from build123d import *

# Parameters (mm, degrees)
F0_W      = 42
F0_H      = 17
F1_DEPTH  = 7
F4_DEPTH  = 25
F5_W      = 42
F5_H      = 5.6745335534
F6_DEPTH  = 10
F7_R      = 1.675
F8_DEPTH  = 25
F9_DEPTH  = 25
F11_W     = 5.7
F11_H     = 7
F12_DEPTH = 5


with BuildPart() as f1:
    # F0 (on Top) → F1 (new body)
    with BuildSketch(Plane.XY):
        with Locations((21, 8.5)):
            Rectangle(F0_W, F0_H)
    extrude(amount=F1_DEPTH)

    # F3 (on face) → F4 (cut)
    with BuildSketch(Plane(origin=(0, 17, 0), x_dir=(-1, 0, 0), z_dir=(0, 1, 0))):
        with BuildLine():
            ThreePointArc((-38.175, 3.5), (-36.5, 1.825), (-34.825, 3.5))
            ThreePointArc((-34.825, 3.5), (-36.5, 5.175), (-38.175, 3.5))
        make_face()
    extrude(amount=-F4_DEPTH, mode=Mode.SUBTRACT)

    # F5 (on face) → F6 (join)
    with BuildSketch(Plane.XY.offset(7)):
        with Locations((21, 14.1627332233)):
            Rectangle(F5_W, F5_H)
    extrude(amount=F6_DEPTH)

    # F7 (on face) → F8 (cut)
    with BuildSketch(Plane(origin=(0, 17, 0), x_dir=(-1, 0, 0), z_dir=(0, 1, 0))):
        with Locations((-36.5, 12.325)):
            Circle(F7_R)
        with Locations((-5.5, 12.325)):
            Circle(F7_R)
    extrude(amount=-F8_DEPTH, mode=Mode.SUBTRACT)

    # F2 (on face) → F9 (cut)
    with BuildSketch(Plane.XY.offset(7)):
        with BuildLine():
            ThreePointArc((16.0693979899, 4.645), (16.0923423463, 4.8945321962), (16.1, 5.145))
            ThreePointArc((16.1, 5.145), (16.0923423463, 5.3954678038), (16.0693979899, 5.645))
            ThreePointArc((16.0693979899, 5.645), (7.9, 5.145), (16.0693979899, 4.645))
        make_face()
        with BuildLine():
            Line((42, 5.145), (16.1, 5.145))
            ThreePointArc((16.1, 5.145), (16.0923423463, 4.8945321962), (16.0693979899, 4.645))
            Line((16.0693979899, 4.645), (42, 4.645))
            Line((42, 4.645), (42, 5.145))
        make_face()
        with BuildLine():
            ThreePointArc((16.0693979899, 5.645), (16.0923423463, 5.3954678038), (16.1, 5.145))
            Line((16.1, 5.145), (42, 5.145))
            Line((42, 5.145), (42, 5.645))
            Line((42, 5.645), (16.0693979899, 5.645))
        make_face()
    extrude(amount=-F9_DEPTH, mode=Mode.SUBTRACT)

    # F11 (on face) → F12 (join)
    with BuildSketch(Plane(origin=(0, 0, 0), x_dir=(0, -1, 0), z_dir=(-1, 0, 0))):
        with Locations((-9.45, 3.5)):
            Rectangle(F11_W, F11_H)
    extrude(amount=F12_DEPTH)


solid = f1.part
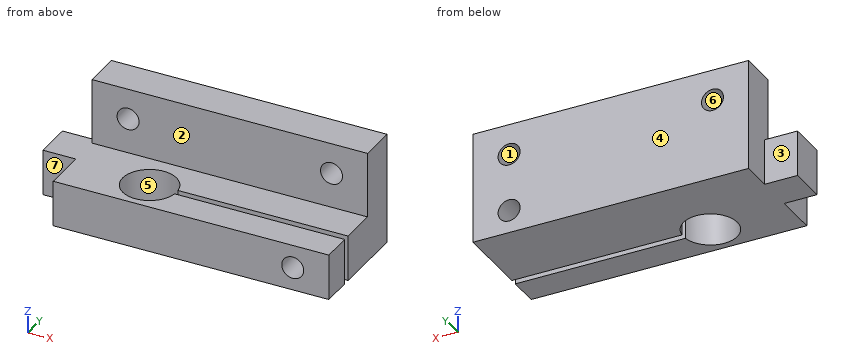
For this review, take the finished solid that the model builds, in its own axes (mm). Face numbers are marked on the shaded views. A direction names the side the tool comes from. Round coordinates to 2 decimals unless told otherwise and drop trailing zeros. Order: outer loops, then holes, each group sorted by start corner. A loop starts at its lowest first (then second) coordinate and runs counter-clockwise, first axis right, second up. Notation, with made-up numbers: M 9,57.5 L 45,57.5 A25 cw 45,83.5 Z; hole C 70,-28 d4. An arc over 180 degrees is marked long. Use a Markdown table: item, result. Add a question column.
Item 1: To check wall thickness, follow line 1 along Z through (x, y) = (36.5, 13) (3 decimals); line 2 along Y through (x, z) = (33, 3.5) (3 decimals); line 3 along Z through (x, y) = (5.5, 13.15). State the ranges of each line that lie inside material, in increasing order.
Item 2: Add section C-C, the plane x = 20. Give the boundary of the cut face in (y, z) (3 decimals).
Item 3: Add section B-B, the plane z = 3.5. Give the boundary of the cut face in (x, y) (3 decimals).
Item 4: Add section D-D, the plane y = 16. Give the boundary of the cut face in (x, z) (3 decimals).
Item 5: Insertion check: pin 1 (4.5 mm diameter, centred on x = 36.5, z = 3.5, fed in from -Y); pin 2 (4 mm diameter, centred on x = -3.5, z = 2, fed in from +Y); pin 3 (3 mm diameter, centred on y = 8, z = 9.5, fed in from +X); pin 4 (4.5 mm diameter, centred on x = 36.5, z = 12.325, fed in from -Y). Each pin has a flat end and moves straight along its axis. Give the tip position at first contact, or say it passes through.
Item 6: Add section A-A, the plane x = 36.5. Give the boundary of the cut face in (y, z) (3 decimals), then the cut area to 3 significant figures.
Item 7: Tool access review of the marked faces 1, 2 and 3: name each direction out of +Z, -Z, +X, -X, +Y, -Y from which nothing blocks a thin tool from reaching the whole face with its end or side.
Item 8: Mouldability with a two-part tool opening along Y and no side actions: class the marked faces 4, 5, 6 and 7 as released by +Y, released by -Y, zero draft, split by the parting line, or undercut.
Geometry results:
| question | item | result |
|---|---|---|
| 1 | line 1 | z = 0 to 1.825, 5.175 to 10.65, 14 to 17 |
| 1 | line 2 | y = 0 to 4.645, 5.645 to 17 |
| 1 | line 3 | z = 0 to 10.65, 14 to 17 |
| 2 | outline | M 0,0 L 4.645,0 L 4.645,7 L 0,7 Z; M 5.645,0 L 17,0 L 17,17 L 11.325,17 L 11.325,7 L 5.645,7 Z |
| 3 | outline | M -5,6.6 L 0,6.6 L 0,0 L 34.825,0 L 34.825,4.645 L 16.069,4.645 A4.1 cw long 16.069,5.645 L 34.825,5.645 L 34.825,17 L 0,17 L 0,12.3 L -5,12.3 Z; M 38.175,0 L 42,0 L 42,4.645 L 38.175,4.645 Z; M 38.175,5.645 L 42,5.645 L 42,17 L 38.175,17 Z |
| 4 | outline | M 0,0 L 42,0 L 42,17 L 0,17 Z; hole C 5.5,12.325 d3.35; hole C 36.5,3.5 d3.35; hole C 36.5,12.325 d3.35 |
| 5 | pin 1 | stops at y = 0 |
| 5 | pin 2 | stops at y = 12.3 |
| 5 | pin 3 | passes through |
| 5 | pin 4 | stops at y = 11.33 |
| 6 | outline | M 0,0 L 4.645,0 L 4.645,1.825 L 0,1.825 Z; M 0,5.175 L 4.645,5.175 L 4.645,7 L 0,7 Z; M 5.645,0 L 17,0 L 17,1.825 L 5.645,1.825 Z; M 5.645,5.175 L 17,5.175 L 17,10.65 L 11.325,10.65 L 11.325,7 L 5.645,7 Z; M 11.325,14 L 17,14 L 17,17 L 11.325,17 Z |
| 6 | area | 96.1 mm² |
| 7 | face 1 | +Y, -Y |
| 7 | face 2 | +Z, +X, -X, -Y |
| 7 | face 3 | +Z, -Z, -X, +Y |
| 8 | face 4 | released by +Y |
| 8 | face 5 | undercut |
| 8 | face 6 | zero draft |
| 8 | face 7 | released by -Y |
